Autodesk Inventor part; units mm, degrees
ref_plane "YZ Plane" through (0, 0, 0) normal (1, 0, 0) x (0, 1, 0)
ref_plane "XZ Plane" through (0, 0, 0) normal (0, 1, 0) x (-1, 0, 0)
ref_plane "XY Plane" through (0, 0, 0) normal (0, 0, 1) x (1, 0, 0)
sketch "Sketch1" plane through (0, 0, 0) normal (0, 0, 1) x (1, 0, 0)
  line L0 (0, 0) -> (69.85, 0)
  line L1 (0, 0) -> (0, 12.7)
  line L2 (95.25, 12.7) -> (69.85, 0)
  line L3 (0, 12.7) -> (-19.05, 12.7)
  line L4 (95.25, 31.75) -> (95.25, 12.7)
  line L5 (-19.05, 44.45) -> (31.75, 44.45)
  line L6 (31.75, 44.45) -> (31.75, 31.75)
  line L7 (31.75, 31.75) -> (95.25, 31.75)
  arc A0 (-48.5968, 56.0712) -> (-19.05, 12.7) centre (-19.05, 44.45) ccw
  line L8 (-19.05, 44.45) -> (-19.05, 95.25)
  line L9 (-19.05, 95.25) -> (-19.05, 101.6)
  arc A1 (-19.05, 114.3) -> (-31.2013, 105.2927) centre (-19.05, 101.6) ccw
  line L10 (-19.05, 101.6) -> (-19.05, 114.3)
  line L11 (-49.3376, 53.975) -> (-30.8232, 106.3625)
  dimension "d0" = 69.85
  dimension "d1" = 12.7
  dimension "d6" = 19.05
  dimension "d17" = 50.8
  dimension "d18" = 12.7
  dimension "d26" = 50.8
  dimension "d29" = 6.35
  dimension "d30" = 25.4
extrude "Extrusion1" add sketch "Sketch1" against normal blind 76.2 contours L1 L3 A0 L11 A1 L10 L9 L8 L5 L6 L7 L4 L2 L0
sketch "Sketch3" plane through (-19.05, 44.45, 0) normal (0, 1, 0) x (1, 0, 0)
  arc A0 (50.8, -0.4913) -> (50.8, 75.7087) centre (50.8, 37.6087) ccw
  line L0 (50.8, 75.7087) -> (50.8, -0.4913)
  line L1 (50.8, 0) -> (50.8, 76.2)
  point P0 (19.05, 0)
  dimension "d40" = 76.2
extrude "Extrusion2" add sketch "Sketch3" against normal up to surface (12.7 mm away)
sketch "Sketch4" plane through (-19.05, 44.45, -76.2) normal (0, 1, 0) x (1, 0, 0)
  point P0 (19.05, -76.2)
  point P1 (50.9967, -38.2666)
hole "Hole2" at (31.9467, 44.45, -37.9334) direction (0, -1, 0) diameter 38.1 end through all
properties part number "Assignment 1.7 - Hanger Jaw"
Input: part model. Units: mm. Frame: model coordinates. A direction names the side the tool comes from. Round coordinates to 2 decimals unless told otherwise and drop trailing zeros. Loops run counter-clockwise (first coordinate to the right, second up) from the corner with the lowest first, then second, coordinate; pieces in that order, holes last. Notation, with made-up numbers: (-32, 77.5) -> (22, 77.5) arc R21 ccw to (22, 103.5) -> close; hole circle Ø2 at (-24, -37). An arc over 180 degrees is marked (long way). Write each question's results on one line, items separated by ' | '.
1. Ray query, line 1 (Y direction, x = 64.5, z = -19.5); line 2 (Z direction, x = 59, y = 8); line 3 (Z direction, x = 42.5, y = 33). Return the intervals inside material, ascending. Write a range as from..to.
Geometry results:
line 1: 0..44.45 | line 2: -76.2..0 | line 3: -74.16..-53.79, -22.07..-1.06
2. First-contact query: P1, Ø5, axis at y = 96.5, z = -26, coming from the +X side; P2, Ø1, axis at x = 65.5, y = 23.5, coming from the +Z side; P3, Ø2, axis at x = -31.5, z = -57.5, coming from the +Y side. Flat tips, straight axial feed; report the tip coordinate or a pass-through.
Geometry results:
P1: x = -19.05 | P2: z = 0 | P3: y = 107.09
3. Section A-A (x = 34). Return loops of the section in (y, z), and give its area (3 significant figures).
Geometry results:
outline: (0, -76.2) -> (31.75, -76.2) -> (31.75, -75.64) -> (44.45, -75.64) -> (44.45, -56.87) -> (0, -56.87) -> close; (0, -18.99) -> (44.45, -18.99) -> (44.45, 0.42) -> (31.75, 0.42) -> (31.75, 0) -> (0, 0) -> close | area: 1,700 mm2
4. Section B-B (y = 41). Return loops of the section in (x, z).
Geometry results:
outline: (-50.61, -76.2) -> (31.75, -76.2) -> (31.75, -75.71) arc R38.1 ccw to (31.75, 0.49) -> (31.75, 0) -> (-50.61, 0) -> close; hole circle Ø38.1 at (31.95, -37.93)
5. Set-up query: faces 1 (the face through (69.84, 38.19, -36.77)), 2 (the face through (0, 6, -38)), 3 (the face through (-19.05, 79, -38)). Return all of +Z, -Z, +X, -X, +Y, -Y with unobstructed straight access to the full face (end or side cutting, diameter ignored); none if empty.
Geometry results:
face 1: +X, +Y | face 2: +Z, -Z, -X, -Y | face 3: +Z, -Z, +X, +Y
6. Section D-D (x = 19). Return loops of the section in (y, z).
Geometry results:
outline: (0, -76.2) -> (44.45, -76.2) -> (44.45, -51.91) -> (0, -51.91) -> close; (0, -23.96) -> (44.45, -23.96) -> (44.45, 0) -> (0, 0) -> close
